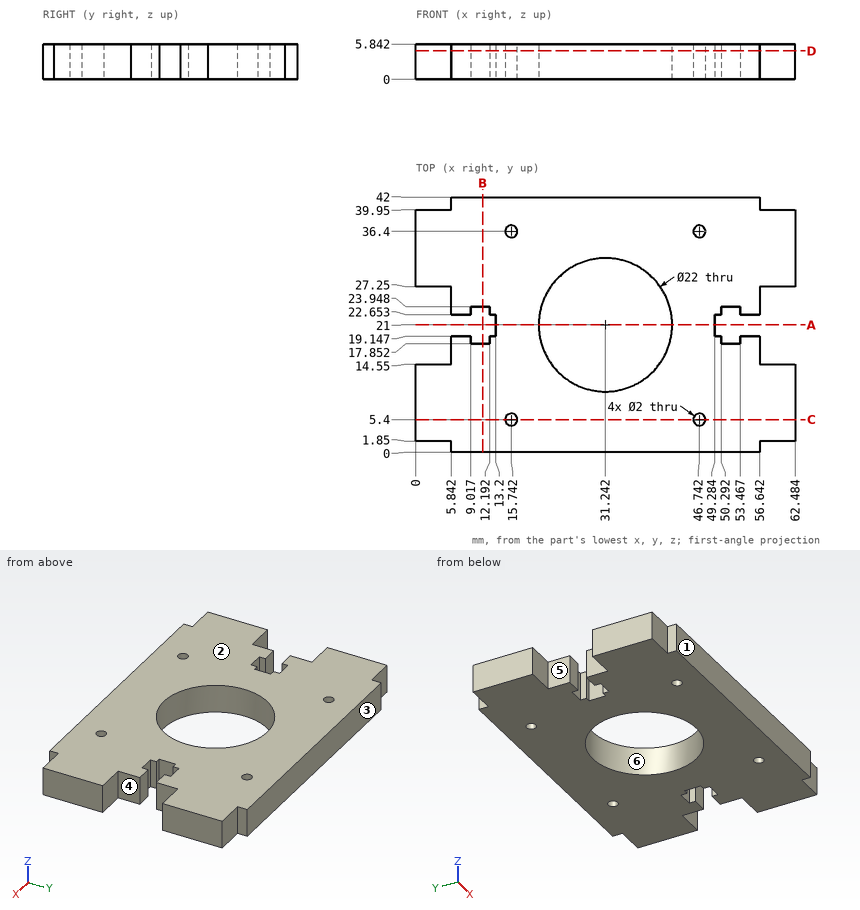
Here's the drawing with two shaded views (mm, measured from the low corner). I have some questions. A direction names the side the tool comes from. Coordinates: 2 decimals unless noted, no trailing zeros. Order: outer loops, then holes, each group sorted by start corner. A loop starts at its lowest first (then second) coordinate and runs counter-clockwise, first axis right, second up. Notation, with made-up numbers: M 40,45.25 L 66,45.25 A13 cw 66,58.25 Z; hole C -17,-18.75 d1. An arc over 180 degrees is marked long. Answer as CSV lines item,"result".
Item 1: We'd pull the mould along Y, two halves only. Please class the marked faces 1, 2, 3 and 4: +Y half, -Y half, draft (parallel to the pull), parting line (faces both ways), or undercut.
Results found:
face 1,"-Y half"
face 2,"draft"
face 3,"+Y half"
face 4,"undercut"
Item 2: Imagine slicing it at C-C on y = 5.4. Write out the boundary of the cut face in (x, z).
Results found:
outline,"M 0,0 L 14.74,0 L 14.74,5.84 L 0,5.84 Z; M 16.74,0 L 45.74,0 L 45.74,5.84 L 16.74,5.84 Z; M 47.74,0 L 62.48,0 L 62.48,5.84 L 47.74,5.84 Z"
Item 3: For pin 1 (3 mm diameter, centred on x = 59, z = 2, fed in from -Y); pin 2 (0.6 mm diameter, centred on y = 23.5, z = 3, fed in from -X); pin 3 (0.6 mm diameter, centred on y = 18.5, z = 2.5, fed in from +X), each with a flat end and sliding along its axis, tell me the tip position at first contact or that it passes through.
Results found:
pin 1,"y = 1.85"
pin 2,"x = 5.84"
pin 3,"x = 56.64"
Item 4: If I drill on line 1 (Y direction, x = 3, z = 1.95); line 2 (Y direction, x = 31, z = 0.55); line 3 (X direction, y = 11, z = 3.1) (1 decimal), over which ranges is the centre line in solid material (lowest first)?
Results found:
line 1,"1.85 to 14.55, 27.25 to 39.95"
line 2,"0 to 10, 32 to 42"
line 3,"0 to 26.7, 35.8 to 62.5"
Item 5: On a 3-axis mill with a long thin cutter (end or side, diameter ignored), from which of +Z, -Z, +X, -X, +Y, -Y can I reach the whole of each face in a straight line? I mean the marked faces 5 and 6. Say none if no direction works.
Results found:
face 5,"+Z, -Z, -X"
face 6,"+Z, -Z"
Item 6: Imagine slicing it at A-A on y = 21. Write out the boundary of the cut face in (x, z).
Results found:
outline,"M 13.2,0 L 20.24,0 L 20.24,5.84 L 13.2,5.84 Z; M 42.24,0 L 49.28,0 L 49.28,5.84 L 42.24,5.84 Z"
Item 7: Imagine slicing it at D-D on z = 4.7. Give the number of separate pieces and of enclosed holes in the cut face, plus the area to 3 significant figures.
Results found:
separate pieces,"1"
enclosed holes,"5"
area,"1,970 mm2"
Item 8: Imagine slicing it at B-B on x = 11. Write out the boundary of the cut face in (y, z), plus the area to 3 significant figures.
Results found:
outline,"M 0,0 L 17.85,0 L 17.85,5.84 L 0,5.84 Z; M 23.95,0 L 42,0 L 42,5.84 L 23.95,5.84 Z"
area,"210 mm2"
